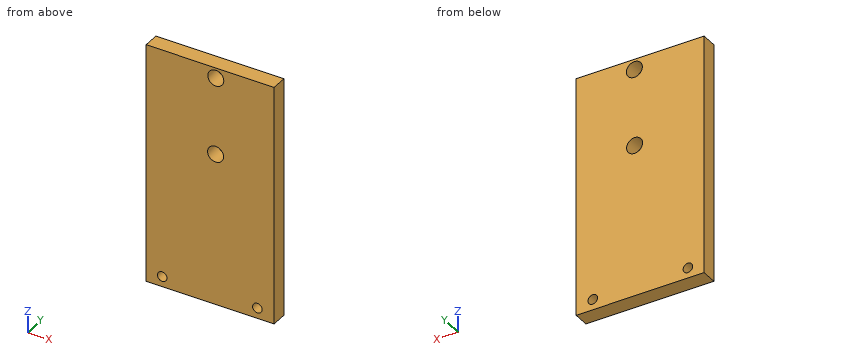
Autodesk Inventor part; units mm, degrees
ref_plane "YZ Plane" through (0, 0, 0) normal (1, 0, 0) x (0, 1, 0)
ref_plane "XZ Plane" through (0, 0, 0) normal (0, 1, 0) x (-1, 0, 0)
ref_plane "XY Plane" through (0, 0, 0) normal (0, 0, 1) x (1, 0, 0)
sketch "Sketch1" plane through (0, 0, 0) normal (0, 1, 0) x (-1, 0, 0)
  line L0 (0, 0) -> (80, 0)
  line L1 (80, 0) -> (80, -150)
  line L2 (80, -150) -> (0, -150)
  line L3 (0, -150) -> (0, 0)
  dimension "d0" = 80
  dimension "d1" = 150
extrude "Extrusion1" add sketch "Sketch1" along normal blind 10
sketch "Sketch2" plane through (0, 0, 0) normal (0, -1, 0) x (1, 0, 0)
  point P0 (0, 0)
  point P1 (-10.4156, -143.4297)
  point P2 (-69.925, -143.618)
hole "Hole1" at (-10.4156, 0, -143.4297) at (-69.925, 0, -143.618) direction (0, 1, 0) diameter 6 end through all
sketch "Sketch3" plane through (0, 0, 0) normal (0, -1, 0) x (1, 0, 0)
  point P0 (0, 0)
  point P1 (-36.5656, -54.7027)
  point P2 (-36.4253, -6.4713)
hole "Hole2" at (-36.5656, 0, -54.7027) at (-36.4253, 0, -6.4713) direction (0, 1, 0) diameter 10 end through all
Model file for the job. Use its own axes, mm. Round coordinates to 2 decimals unless told otherwise and drop trailing zeros. Loops run counter-clockwise (first coordinate to the right, second up) from the corner with the lowest first, then second, coordinate; pieces in that order, holes last.
1. Band-saw the part on B-B, the plane z = -54.5. List the corners of the cut face in (x, y).
Check values:
outline: (-80, 0) - (-41.56, 0) - (-41.56, 10) - (-80, 10) - close; (-31.57, 0) - (0, 0) - (0, 10) - (-31.57, 10) - close
2. Band-saw the part on A-A, the plane y = 2. List the corners of the cut face in (x, z) (3 decimals), and give its area (3 significant figures).
Check values:
outline: (-80, -150) - (0, -150) - (0, 0) - (-80, 0) - close; hole circle Ø6 at (-69.925, -143.618); hole circle Ø10 at (-36.566, -54.703); hole circle Ø10 at (-36.425, -6.471); hole circle Ø6 at (-10.416, -143.43)
area: 11,800 mm2
3. Drop a flat-ended pin along its axis: P1, Ø8, axis at x = -36.43, z = -6.47, coming from the -Y side. Give the stop position or say it passes through.
Check values:
P1: passes through
4. Wall check: probe 1 along Z at (x, y) = (-36.5, 5); probe 2 along Z at (x, y) = (-70, 5); probe 3 along X at (y, z) = (5.25, -50.5). Give the ranges that are in metal, low to high.
Check values:
probe 1: z = -150 to -59.7, -49.7 to -11.47, -1.47 to 0
probe 2: z = -150 to -146.62, -140.62 to 0
probe 3: x = -80 to -39.27, -33.86 to 0
